Build history of the part. All positions in model axes, mm. Face numbers are marked on the shaded views. A direction names the side the tool comes from. Coordinates: 2 decimals unless noted, no trailing zeros. Loops run counter-clockwise (first coordinate to the right, second up) from the corner with the lowest first, then second, coordinate; pieces in that order, holes last. Notation, with made-up numbers: M 49.25,20 L 81.25,20 A18 ccw 81.25,52 Z; hole C 51,49 d3. An arc over 180 degrees is marked long. Write each question's results on one line, items separated by ' | '. Start each with the question number.
from build123d import *

# Parameters (mm, degrees)
F0_R     = 18
F1_DEPTH = 33


with BuildPart() as f1:
    # F0 (on Top) → F1 (new body)
    with BuildSketch(Plane.XY):
        Circle(F0_R)
        with BuildLine():
            ThreePointArc((-5.7976616963, 1.9755363461), (1.0012360136, 6.0426113101), (6.125, 0))
            ThreePointArc((6.125, 0), (1.0012360136, -6.0426113101), (-5.7976616963, -1.9755363461))
            Line((-5.7976616963, -1.9755363461), (-5.7976616963, -2.0244636539))
            Line((-5.7976616963, -2.0244636539), (-17.8778566858, -2.0244636539))
            Line((-17.8778566858, -2.0244636539), (-17.8778566858, 1.9755363461))
            Line((-17.8778566858, 1.9755363461), (-5.7976616963, 1.9755363461))
        make_face(mode=Mode.SUBTRACT)
    extrude(amount=F1_DEPTH)


solid = f1.part
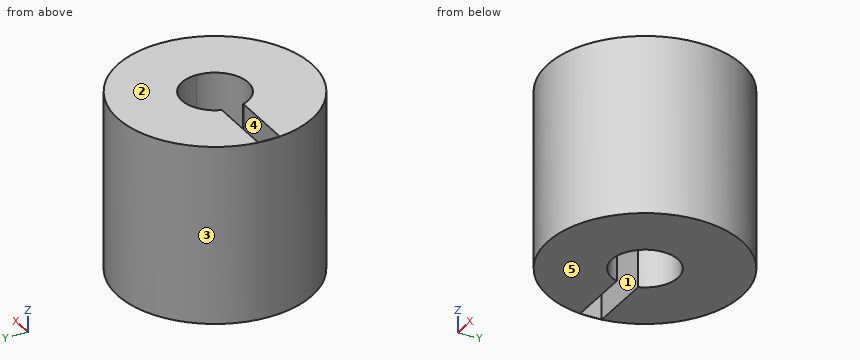
1. Which spindle directions (+Z, -Z, +X, -X, +Y, -Y) get a long thin tool onto all of the face, cutting with end or side? Do the marked faces 1 and 2. Say none if no direction does.
2. Mould opens along Y. For the marked faces 3, 4 and 5 say: +Y half, -Y half, draft (parallel to the pull), parting line (faces both ways), or undercut.
3. Band-saw the part on D-D, the plane x = 8.5. List the corners of the cut face in (y, z).
4. Pin check, flat tips, straight feed: pin 1 (1.2 mm diameter, centred on y = 1, z = 21.5, fed in from +X); pin 2 (10 mm diameter, centred on y = 11, z = 12.5, fed in from +X); pin 3 (1.5 mm diameter, centred on y = -13, z = 23.5, fed in from -X); pin 4 (12 mm diameter, centred on y = 4, z = 18.5, fed in from -X). Stop position of each tip, or through.
5. Band-saw the part on C-C, the plane y = -1. List the corners of the cut face in (x, z).
6. Wall check: line 1 along Y through (x, z) = (-12, 22); line 2 along Y through (x, z) = (-14, 9.5); line 3 along X through (y, z) = (4.5, 12). Give the ranges that are in metal, low to high.
7. Band-saw the part on A-A, the plane z = 16. List the corners of the cut face in (x, y) (3 decimals).
8. Band-saw the part on B-B, the plane x = 0. List the corners of the cut face in (y, z) (3 decimals), plus the area to 3 significant figures.
Checked values:
1) face 1: +Z, -Z | face 2: +Z, +X, -X, +Y, -Y
2) face 3: parting line | face 4: undercut | face 5: draft
3) outline: M -15.87,0 L 15.87,0 L 15.87,33 L -15.87,33 Z
4) pin 1: x = 18 | pin 2: x = 16.97 | pin 3: x = -13.19 | pin 4: x = -18
5) outline: M -17.97,0 L -17.88,0 L -17.88,33 L -17.97,33 Z; M 6.04,0 L 17.97,0 L 17.97,33 L 6.04,33 Z
6) line 1: -13.42 to -2.02, 1.98 to 13.42 | line 2: -11.31 to -2.02, 1.98 to 11.31 | line 3: -17.43 to -4.16, 4.16 to 17.43
7) outline: C 0,0 d36; hole M -17.878,-2.024 L -5.798,-2.024 L -5.798,-1.976 A6.125 ccw long -5.798,1.976 L -17.878,1.976 Z
8) outline: M -18,0 L -6.125,0 L -6.125,33 L -18,33 Z; M 6.125,0 L 18,0 L 18,33 L 6.125,33 Z | area: 784 mm²
